```python
from build123d import *

# Parameters (mm, degrees)
F2_SIZE = 1


# Not quite as in the source:
# - a fillet or chamfer that OpenCascade refuses, or shapes differently, is made with other operations: its cross-section is extruded or revolved along the edge and cut away or added


with BuildPart() as f1:
    # F0 (on Front) → F1 (revolve)
    with BuildSketch(Plane.XZ):
        with BuildLine():
            Line((-5.2, 0), (-5.2, 20.18))
            Line((-5.2, 20.18), (-14, 20.18))
            ThreePointArc((-14, 20.18), (-11.0994378784, 10.09), (-14, 0))
            Line((-14, 0), (-5.2, 0))
        make_face()
    revolve(axis=Axis((0, 0, 10.09), (0, 0, 1)))

    # F2
    f2_edges = [f1.edges().sort_by_distance(p)[0] for p in [
        (5.2, 0, 0),
        (5.2, 0, 20.18),
        (-5.2, 0, 10.09),
    ]]
    chamfer(f2_edges, length=F2_SIZE)

    # F3: chamfer of 2 on 3 edges, made by hand

    # F3_s1 → F3_t2 (revolve, cut)
    with BuildSketch(Plane.XZ):
        with BuildLine():
            Line((-13.1431767576, 18.5105716839), (-12.0687646644, 20.2480416136))
            Line((-12.0687646644, 20.2480416136), (-12.0687646644, 20.2880416136))
            ThreePointArc((-12.0687646644, 20.2880416136), (-13.0343823322, 20.22), (-14, 20.22))
            Line((-14, 20.22), (-14.0338935534, 20.1587578947))
            ThreePointArc((-14.0338935534, 20.1587578947), (-13.556591594, 19.3536837603), (-13.1789627292, 18.4927009191))
            Line((-13.1789627292, 18.4927009191), (-13.1431767576, 18.5105716839))
        make_face()
    revolve(axis=Axis((0, 0, 20.18), (0, 0, 1)), mode=Mode.SUBTRACT)

    # F3_s3 → F3_t4 (revolve, cut)
    with BuildSketch(Plane.XZ):
        with BuildLine():
            Line((-12.0687646644, -0.0680416136), (-13.1431767576, 1.6694283161))
            Line((-13.1431767576, 1.6694283161), (-13.1789627292, 1.6872990809))
            ThreePointArc((-13.1789627292, 1.6872990809), (-13.556591594, 0.8263162397), (-14.0338935534, 0.0212421053))
            Line((-14.0338935534, 0.0212421053), (-14, -0.04))
            ThreePointArc((-14, -0.04), (-13.0343823322, -0.04), (-12.0687646644, -0.1080416136))
            Line((-12.0687646644, -0.1080416136), (-12.0687646644, -0.0680416136))
        make_face()
    revolve(axis=Axis((0, 0, 0), (0, 0, 1)), mode=Mode.SUBTRACT)


solid = f1.part
```
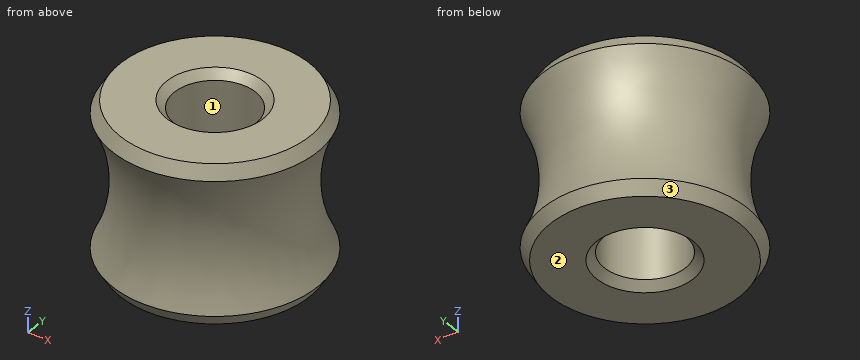
Verification items for the finished model (mm, model axes). Face numbers are marked on the shaded views. Give positions to 0.01 mm unless a question says otherwise; leave off trailing zeros. Write each loop counter-clockwise with the first axis right and the second up, starting at its lowest first coordinate (ties: lowest second). Pieces come first, ordered by that corner, then holes. Notation, with made-up numbers: M 49,79 L 96,79 A25 cw 96,108 Z; hole C 58,-12 d5. An arc over 180 degrees is marked long. One line per question, with ' | ' between items.
1) Section check C-C on z = 14.75. Enter the section's corners in (x, y).
Result:
outline: C 0,0 d23.36; hole C 0,0 d10.4
2) Section check A-A on y = 0. Enter the section's corners in (x, z), plus the area to 3 significant figures.
Result:
outline: M -13.1,1.6 L -12.11,0 L -6.2,0 L -5.2,1 L -5.2,19.18 L -6.2,20.18 L -12.11,20.18 L -13.1,18.58 A19 cw Z; M 5.2,1 L 6.2,0 L 12.11,0 L 13.1,1.6 A19 cw 13.1,18.58 L 12.11,20.18 L 6.2,20.18 L 5.2,19.18 Z | area: 268 mm2
3) Gauge pin test, flat ends, axial feed: pin 1 Ø2 at (x, z) = (-10, 10) entering from -Y; pin 2 Ø1 at (x, z) = (4.5, 14) entering from +Y; pin 3 Ø12 at (x, y) = (0.5, 3.5) entering from -Z; pin 4 Ø2 at (x, y) = (1, 4.5) entering from -Z. Record the tip position at first contact, or that the pin passes through.
Result:
pin 1: stops at y = -6.5 | pin 2: stops at y = 10.82 | pin 3: stops at z = 0 | pin 4: stops at z = 0.59
4) Thickness scan on line 1 along Y through (x, z) = (0, 9.25); line 2 along X through (y, z) = (-1.25, 11.75); line 3 along X through (y, z) = (1.5, 13). Record the ranges inside material, lowest first. Write a range as [from, to].
Result:
line 1: y = [-11.12, -5.2], [5.2, 11.12] | line 2: x = [-11.1, -5.05], [5.05, 11.1] | line 3: x = [-11.22, -4.98], [4.98, 11.22]
5) Mould release check, pull along Y, two halves, no side actions. Record for the marked faces 1, 2 and 3: released by +Y, released by -Y, zero draft, split by the parting line, or undercut.
Result:
face 1: undercut | face 2: zero draft | face 3: split by the parting line
6) Section check D-D on z = 3.25. Enter the section's corners in (x, y), plus the area to 3 significant figures.
Result:
outline: C 0,0 d24.75; hole C 0,0 d10.4 | area: 396 mm2
